Autodesk Inventor part; units mm, degrees
ref_plane "YZ Plane" through (0, 0, 0) normal (1, 0, 0) x (0, 1, 0)
ref_plane "XZ Plane" through (0, 0, 0) normal (0, 1, 0) x (-1, 0, 0)
ref_plane "XY Plane" through (0, 0, 0) normal (0, 0, 1) x (1, 0, 0)
sketch "スケッチ1" plane through (0, 0, 0) normal (1, 0, 0) x (0, 1, 0)
  circle A0 centre (0, 0) radius 3.55
  arc A1 (4.3581, -2.4508) -> (0, 5) centre (0, 0) ccw
  line L0 (4.3581, -2.4508) -> (-1.5743, -13)
  line L1 (-1.5743, -13) -> (-6, -13)
  line L2 (-6, -13) -> (-6, 5)
  line L3 (-6, 5) -> (0, 5)
  circle A2 centre (0, 0) radius 3
  dimension "d0" = 7.1
  dimension "d1" = 5
  dimension "d2" = 18
  dimension "d3" = 6
  dimension "d6" = 6
extrude "押し出し1" add sketch "スケッチ1" along normal blind 3 contours A0 | L0 L1 L2 L3 A1
extrude "押し出し2" cut sketch "スケッチ1" along normal blind 0.8 contours A0 | A2
properties part number "Stand"
Could you check a few things on this model? Use its own coordinates, in mm. A direction names the side the tool comes from. Coordinates: 2 decimals unless noted, no trailing zeros. Write each loop counter-clockwise with the first axis right and the second up, starting at its lowest first coordinate (ties: lowest second). Pieces come first, ordered by that corner, then holes. Notation, with made-up numbers: (2.25, 63) -> (37.25, 63) arc R19 ccw to (37.25, 98) -> close; hole circle Ø4 at (13, -36). An arc over 180 degrees is marked (long way). Write item = value, one per line. Start each with the question number.
(1) I want a section at C-C (y = 0.5). Please give me the cut outline in (x, z).
(2) We'd pull the mould along Z, two halves only. Please class faces 1 (the face through (1, -6, -4)), 2 (the face through (2, -3, 0)), 3 (the face through (1.479, 1.433, -7.652)), 4 (the face through (0.8, -1, 3)): released by +Z, released by -Z, zero draft, split by the parting line, or undercut.
(3) I want a section at B-B (x = 1.4). Please give me the cut outline in (y, z).
(4) Will these pins go through, and if not, where does the flat tip stop? pin 1 (1.5 mm diameter, centred on x = 1.5, y = 3, fed in from -Z); pin 2 (3.5 mm diameter, centred on y = 0, z = -1.5, fed in from -X); pin 3 (2 mm diameter, centred on y = 1, z = -8, fed in from -X).
(5) Which directions (+Z, -Z, +X, -X, +Y, -Y) give clear straight access to the entire face, cutting with the end or side of a thin tool? Please do faces 5 (the face through (1, -3, 5)), 6 (the face through (0.39, -0.46, -3.52)).
(6) I want a section at A-A (z = 0). Please give me the cut outline in (x, y), plus the area to 3 significant figures.
(7) I want a section at D-D (z = -3.25). Please give me the cut outline in (x, y).
(8) I need wall thicknesses on line 1 (Y direction, x = 1.5, z = 0); line 2 (Z direction, x = 0.45, y = 0); line 3 (Z direction, x = 2.2, y = 0). Which ranges of each line are inside material? Lowest first, please. Write a range as [from, to].
Result set:
q1.outline = (0, -9.31) -> (3, -9.31) -> (3, -2.96) -> (0.8, -2.96) -> (0.8, -3.51) -> (0, -3.51) -> close; (0, 3.51) -> (0.8, 3.51) -> (0.8, 2.96) -> (3, 2.96) -> (3, 4.97) -> (0, 4.97) -> close
q2.face_1 = zero draft
q2.face_2 = undercut
q2.face_3 = released by -Z
q2.face_4 = undercut
q3.outline = (-6, -13) -> (-1.57, -13) -> (4.36, -2.45) arc R5 ccw to (0, 5) -> (-6, 5) -> close; hole circle Ø6 at (0, 0)
q4.pin_1 = -6.2
q4.pin_2 = 0.8
q4.pin_3 = 0
q5.face_5 = +Z, +X, -X, +Y, -Y
q5.face_6 = -X
q6.outline = (0, -6) -> (3, -6) -> (3, -3) -> (0.8, -3) -> (0.8, -3.55) -> (0, -3.55) -> close; (0, 3.55) -> (0.8, 3.55) -> (0.8, 3) -> (3, 3) -> (3, 5) -> (0, 5) -> close
q6.area = 14.1 mm2
q7.outline = (0, -6) -> (3, -6) -> (3, 3.91) -> (0, 3.91) -> (0, 1.43) -> (0.8, 1.43) -> (0.8, -1.43) -> (0, -1.43) -> close
q8.line_1 = [-6, -3], [3, 5]
q8.line_2 = [-10.2, -3.55], [3.55, 5]
q8.line_3 = [-10.2, -3], [3, 5]
